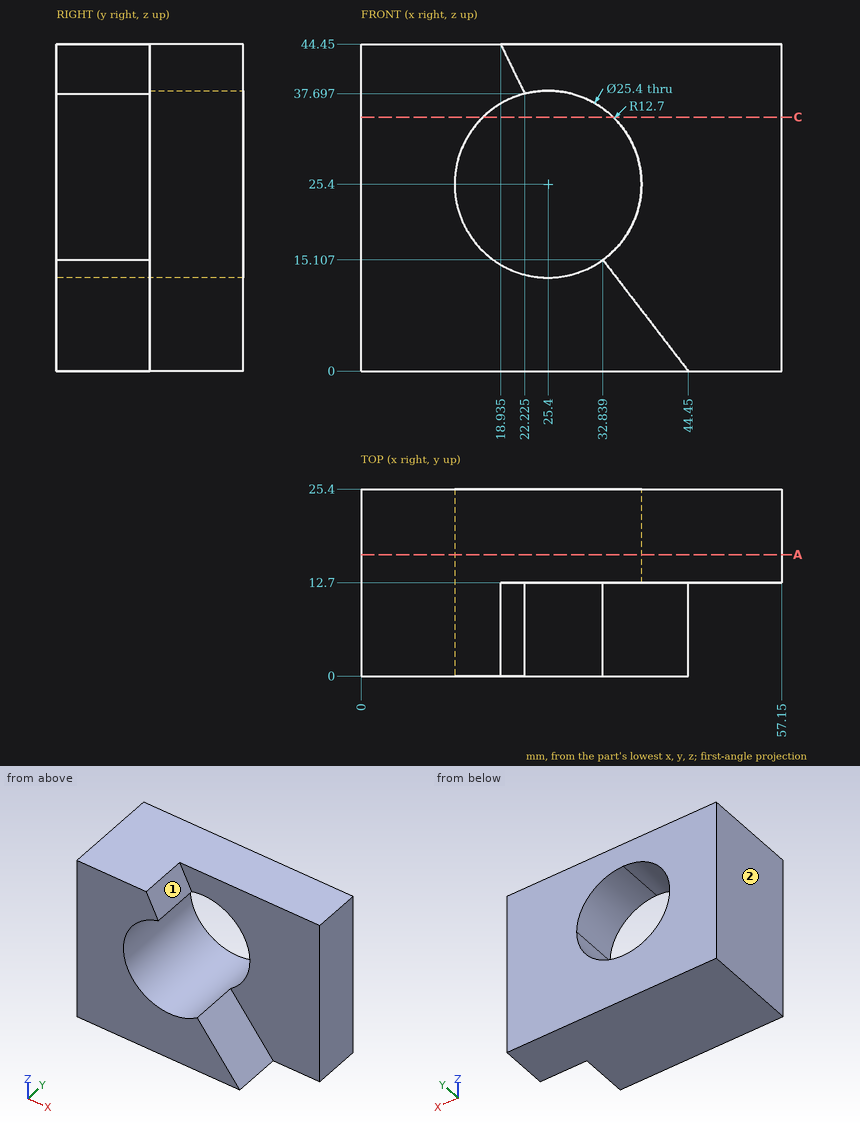
Here's the drawing with two shaded views (mm, measured from the low corner). I have some questions. A direction names the side the tool comes from. Coordinates: 2 decimals unless noted, no trailing zeros. Loops run counter-clockwise (first coordinate to the right, second up) from the corner with the lowest first, then second, coordinate; pieces in that order, holes last. Notation, with made-up numbers: (54, -19.75) -> (104, -19.75) arc R13 cw to (104, -12.75) -> close; hole circle Ø10 at (30, 2.5). An arc over 180 degrees is marked (long way). Put each result on its own line as item: value. Start each with the question number.
Q1. I want a section at A-A (y = 16.5). Write out the boundary of the cut face in (x, z), plus the area to 3 significant figures.
Q2. For the marked faces 1 and 2, which set-ups out of +Z, -Z, +X, -X, +Y, -Y let a thin tool reach every point of the face, with its end or its side?
Q3. If I drill on line 1 (X direction, y = 16, z = 25.4); line 2 (Z direction, x = 25.4, y = 14); line 3 (Y direction, x = 39.5, z = 8.5), over which ranges is the centre line in solid material (lowest first)? Write a range as [from, to].
Q4. I want a section at C-C (z = 34.5). Write out the boundary of the cut face in (x, y).
Q5. I'm going to push flat-ended pins straight in: P1, Ø5, axis at y = 6.5, z = 12.5, coming from the +X side (1 decimal); P2, Ø1.5, axis at x = 45.5, z = 37.5, coming from the -Y side. Where does each tip first touch, or does it pass through?
Taken from the geometry:
1. outline: (0, 0) -> (57.15, 0) -> (57.15, 44.45) -> (0, 44.45) -> close; hole circle Ø25.4 at (25.4, 25.4)
1. area: 2,030 mm2
2. face 1: +Z, +X, -Y
2. face 2: +Z, -Z, -X, +Y, -Y
3. line 1: x = [0, 12.7], [38.1, 57.15]
3. line 2: z = [0, 12.7], [38.1, 44.45]
3. line 3: y = [12.7, 25.4]
4. outline: (0, 0) -> (16.54, 0) -> (16.54, 25.4) -> (0, 25.4) -> close; (34.26, 12.7) -> (57.15, 12.7) -> (57.15, 25.4) -> (34.26, 25.4) -> close
5. P1: stops at x = 36.8
5. P2: stops at y = 12.7
